from build123d import *

# Parameters (mm, degrees)
SKETCH8_W                          = 5
SKETCH8_H                          = 46.4
BOSS_EXTRUDE6_DEPTH                = 13.9
SKETCH9_W                          = 5
SKETCH9_H                          = 46.4
BOSS_EXTRUDE7_DEPTH                = 131
SKETCH11_W                         = 16.3
SKETCH11_H                         = 10.35
BOSS_EXTRUDE8_DEPTH                = 5
SKETCH10_R                         = 5.5
SKETCH10_R_2                       = 3.15
CUT_EXTRUDE2_DEPTH                 = 5
SKETCH16_R                         = 4.7625
CUT_EXTRUDE6_DEPTH                 = 9
SKETCH17_R                         = 3.5
CUT_EXTRUDE7_DEPTH                 = 9
M2_5X0_45_TAPPED_HOLE1_D           = 2.05
M2_5X0_45_TAPPED_HOLE1_DEPTH       = 12.5
M2_5X0_45_TAPPED_HOLE1_CSINK_D     = 2.55
M2_5X0_45_TAPPED_HOLE1_CSINK_ANGLE = 90
M2_5X0_45_TAPPED_HOLE1_TIP         = 0.615882135


with BuildPart() as part:
    # Sketch8 → Boss-Extrude6 (new body)
    with BuildSketch(Plane(origin=(0, 0, 0), x_dir=(0, 0, -1), z_dir=(1, 0, 0))):
        with Locations((65.5, 47)):
            Rectangle(SKETCH8_W, SKETCH8_H)
    extrude(amount=BOSS_EXTRUDE6_DEPTH)

    # Sketch9 → Boss-Extrude7 (add)
    with BuildSketch(Plane(origin=(0, 0, -68), x_dir=(-1, 0, 0), z_dir=(0, 0, -1))):
        with Locations((-11.4, 47)):
            Rectangle(SKETCH9_W, SKETCH9_H)
    extrude(amount=BOSS_EXTRUDE7_DEPTH)

    # Sketch11 → Boss-Extrude8 (add)
    with BuildSketch(Plane(origin=(13.9, 0, 0), x_dir=(0, 0, -1), z_dir=(1, 0, 0))):
        with Locations((116.5, 75.375)):
            Rectangle(SKETCH11_W, SKETCH11_H)
    extrude(amount=-BOSS_EXTRUDE8_DEPTH)

    # Sketch10 → Cut-Extrude2 (cut)
    with BuildSketch(Plane(origin=(13.9, 0, 0), x_dir=(0, 0, -1), z_dir=(1, 0, 0))):
        with Locations((116.5, 47)):
            Circle(SKETCH10_R)
        with Locations((116.5, 72.4)):
            Circle(SKETCH10_R_2)
        with Locations((138.497045256, 34.3)):
            Circle(SKETCH10_R_2)
        with Locations((94.502954744, 34.3)):
            Circle(SKETCH10_R_2)
    extrude(amount=-CUT_EXTRUDE2_DEPTH, mode=Mode.SUBTRACT)

    # Sketch16 → Cut-Extrude6 (cut)
    with BuildSketch(Plane(origin=(13.9, 0, 0), x_dir=(0, 0, -1), z_dir=(1, 0, 0))):
        with Locations((180.348526442, 49.5625)):
            Circle(SKETCH16_R)
    extrude(amount=-CUT_EXTRUDE6_DEPTH, mode=Mode.SUBTRACT)

    # Sketch17 → Cut-Extrude7 (cut)
    with BuildSketch(Plane(origin=(13.9, 0, 0), x_dir=(0, 0, -1), z_dir=(1, 0, 0))):
        with Locations((162.886026442, 49.5625)):
            Circle(SKETCH17_R)
    extrude(amount=-CUT_EXTRUDE7_DEPTH, mode=Mode.SUBTRACT)

    # M2.5x0.45 Tapped Hole1
    with Locations(Plane.ZY):
        with Locations((-65.5, 62), (-65.5, 52), (-65.5, 32), (-65.5, 42)):
            CounterSinkHole(M2_5X0_45_TAPPED_HOLE1_D / 2, M2_5X0_45_TAPPED_HOLE1_CSINK_D / 2, depth=M2_5X0_45_TAPPED_HOLE1_DEPTH, counter_sink_angle=M2_5X0_45_TAPPED_HOLE1_CSINK_ANGLE)
            with Locations((0, 0, -(M2_5X0_45_TAPPED_HOLE1_DEPTH + M2_5X0_45_TAPPED_HOLE1_TIP / 2))):  # 118° drill point
                Cone(0, M2_5X0_45_TAPPED_HOLE1_D / 2, M2_5X0_45_TAPPED_HOLE1_TIP, mode=Mode.SUBTRACT)


solid = part.part
Could you check a few things on this model? Use its own coordinates, in mm. A direction names the side the tool comes from. Give positions to 0.01 mm unless a question says otherwise; leave off trailing zeros. Write each loop counter-clockwise with the first axis right and the second up, starting at its lowest first coordinate (ties: lowest second). Pieces come first, ordered by that corner, then holes. Notation, with made-up numbers: (-8, -12.5) -> (30, -12.5) arc R22 ccw to (30, 16.5) -> close; hole circle Ø6 at (36, 12.5). An arc over 180 degrees is marked (long way). Write each question's results on one line, items separated by ' | '. Start each with the question number.
Q1. Suppose I cut it at C-C, the plane y = 67. List the corners of the cut face in (x, z) for me, and give its area (4 significant figures).
Q2. Suppose I cut it at B-B, the plane x = 1.5. List the corners of the cut face in (y, z) for me (3 decimals), and give its area (3 significant figures).
Q3. Suppose I cut it at A-A, the plane z = -116.5. List the corners of the cut face in (x, y) for me, and give its area (3 significant figures).
Q4. We'd pull the mould along Z, two halves only. Please class faces 4 (the face through (7, 47, -63)), 5 (the face through (11.44, 74.53, -114.18)), 6 (the face through (4, 47, -68)), 7 (the face through (8.9, 45, -133)): +Z half, -Z half, draft (parallel to the pull), parting line (faces both ways), or undercut.
Q5. Which directions (+Z, -Z, +X, -X, +Y, -Y) give clear straight access to the entire face, cutting with the end or side of a thin tool? Please do faces 1 (the face through (11.435, 50.614, -166.224)), 2 (the face through (11, 75, -108.35)), 3 (the face through (11, 75, -124.65)).
Q6. I'm going to push flat-ended pins straight in: pin 1 Ø5.5 at (x, y) = (11.5, 78) entering from +Z; pin 2 Ø2.5 at (x, y) = (4.5, 55) entering from -Z; pin 3 Ø2 at (y, z) = (62, -107.5) entering from -X. Where does each tip first touch, or does it pass through?
Q7. I need wall thicknesses on probe 1 along Y at (x, z) = (7.5, -65.5) (3 decimals); probe 2 along Z at (x, y) = (9.25, 62) (3 decimals); probe 3 along Y at (x, z) = (12.55, -116.5). Which ranges of each line are inside material? Lowest first, please.
Q8. Suppose I cut it at D-D, the plane x = 11.25. State how many separate pieces and enclosed holes the cut face has, and give its area (3 significant figures).
Outcome:
1) outline: (0, -68) -> (8.9, -68) -> (8.9, -199) -> (13.9, -199) -> (13.9, -63) -> (0, -63) -> close | area: 724.5 mm2
2) outline: (23.8, -68) -> (70.2, -68) -> (70.2, -63) -> (23.8, -63) -> close; hole circle Ø2.05 at (32, -65.5); hole circle Ø2.05 at (42, -65.5); hole circle Ø2.05 at (52, -65.5); hole circle Ø2.05 at (62, -65.5) | area: 219 mm2
3) outline: (8.9, 23.8) -> (13.9, 23.8) -> (13.9, 41.5) -> (8.9, 41.5) -> close; (8.9, 52.5) -> (13.9, 52.5) -> (13.9, 69.25) -> (8.9, 69.25) -> close; (8.9, 75.55) -> (13.9, 75.55) -> (13.9, 80.55) -> (8.9, 80.55) -> close | area: 197 mm2
4) face 4: +Z half | face 5: undercut | face 6: -Z half | face 7: draft
5) face 1: +X, -X | face 2: +Z, +X, -X, +Y | face 3: -Z, +X, -X, +Y
6) pin 1: z = -108.35 | pin 2: z = -68 | pin 3: x = 8.9
7) probe 1: 23.8 to 30.975, 33.025 to 40.975, 43.025 to 50.975, 53.025 to 60.975, 63.025 to 70.2 | probe 2: -199 to -66.525, -64.475 to -63 | probe 3: 23.8 to 41.5, 52.5 to 69.25, 75.55 to 80.55
8) separate pieces: 1 | enclosed holes: 10 | area: 6,170 mm2
